Source: CAD feature listing. Evaluate the final solid. Frame: model axes, mm. A direction names the side the tool comes from. Give positions to 0.01 mm unless a question says otherwise; leave off trailing zeros. Write each loop counter-clockwise with the first axis right and the second up, starting at its lowest first coordinate (ties: lowest second). Pieces come first, ordered by that corner, then holes. Notation, with made-up numbers: (-31, 60) - (-6, 60) arc R26 ccw to (-6, 95) - close; hole circle Ø9 at (35.25, -23). An arc over 180 degrees is marked (long way). One line per question, with ' | ' between items. Start each with the question number.
(1) Access query for faces 1 (the cylindrical face through (160.406, 19.977, 33.495)), 2 (the cylindrical face through (160.406, -38.996, 0.554)), 3 (the cylindrical face through (158, 22, -29)). Directions: +Z, -Z, +X, -X, +Y, -Y. A direction counts if a zero-diameter tool reaches every point of the face in a straight line with its end or side. Return the directions, or none.
(2) Section B-B, the plane y = 0. Return loops of the section in (x, z).
(3) Section D-D, the plane x = 154. Return loops of the section in (y, z), plus the area to 3 significant figures.
(4) Section A-A, the plane z = 0. Return loops of the section in (x, y), plus the area to 3 significant figures.
(5) Ray query, line 1 (Y direction, x = 164, z = 0); line 2 (X direction, y = -5.5, z = -31); line 3 (Z direction, x = 163.5, y = -24.5). Return the intervals inside material, ascending. Write a range as [from, to].
(6) Draft query along Z for faces 4 (the cylindrical face through (160.406, 19.019, -34.048)), 5 (the flat face through (139.7, 38.02, -9.35)), 6 (the cylindrical face through (153.267, -18.922, -33.391)), 7 (the cylindrical face through (180.71, 20.76, 10.8)). Return one class per face: +Z half, -Z half, draft (parallel to the pull), parting line (faces both ways), or undercut.
(7) Section C-C, the plane z = 14.5. Return loops of the section in (x, y), plus the area to 3 significant figures.
(8) Pin query (flat end, axial travel): pin 1 (12 mm diameter, centred on x = 168.5, y = 6.5, fed in from -Z); pin 2 (1.5 mm diameter, centred on x = 144, y = 30, fed in from +Z); pin 3 (12 mm diameter, centred on x = 150, z = 16.5, fed in from -Y). Return the tip coordinate at first contact, or that it passes through.
```python
from build123d import *

# Parameters (mm, degrees)
AXIAL_HOLES_DEPTH      = 192.606080279
AXIAL_HOLES_DEPTH_BACK = 192.606080279
SKETCH2_R              = 1.65


with BuildPart() as part:
    # Axial profile (mm) → Full revolution (revolve)
    with BuildSketch(Plane.XY, mode=Mode.PRIVATE) as full_revolution_sk:
        Polygon((135.7, 36.4), (179.7, 36.4), (179.7, 23.4), (181.7, 23.4), (181.7, 39), (139.7, 39), (139.7, 43), (135.7, 43), align=None)
    revolve(full_revolution_sk.sketch.rotate(Axis((-110, 0, 0), (1, 0, 0)), 90), axis=Axis((-110, 0, 0), (1, 0, 0)))

    # Sketch2 → Axial holes (cut, two sides: drawn at the far end of the back side and taken through both)
    with BuildSketch(Plane(origin=(0, 0, 0), x_dir=(0, 0, -1), z_dir=(1, 0, 0)).offset(-AXIAL_HOLES_DEPTH_BACK)):
        with Locations(Location((0, 40, 0), (0, 0, 218.251159994))):
            Circle(SKETCH2_R)
        with Locations(Location((-34.641016151, -20, 0), (0, 0, 81.748840006))):
            Circle(SKETCH2_R)
        with Locations(Location((34.641016151, -20, 0), (0, 0, 201.748840006))):
            Circle(SKETCH2_R)
    extrude(amount=AXIAL_HOLES_DEPTH + AXIAL_HOLES_DEPTH_BACK, mode=Mode.SUBTRACT)


solid = part.part
```
Check sheet entries:
1) face 1: +Z, +X | face 2: +X, -Y | face 3: -X
2) outline: (135.7, -43) - (139.7, -43) - (139.7, -39) - (181.7, -39) - (181.7, -23.4) - (179.7, -23.4) - (179.7, -36.4) - (135.7, -36.4) - close; (135.7, 36.4) - (179.7, 36.4) - (179.7, 23.4) - (181.7, 23.4) - (181.7, 39) - (139.7, 39) - (139.7, 43) - (135.7, 43) - close
3) outline: (-20.61, -33.11) arc R1.65 cw to (-18.37, -34.4) arc R39 ccw to (38.98, -1.3) arc R1.65 cw to (38.98, 1.3) arc R39 ccw to (-18.37, 34.4) arc R1.65 cw to (-20.61, 33.11) arc R39 ccw to start; hole circle Ø72.8 at (0, 0) | area: 612 mm²
4) outline: (135.7, -43) - (139.7, -43) - (139.7, -39) - (181.7, -39) - (181.7, -23.4) - (179.7, -23.4) - (179.7, -36.4) - (135.7, -36.4) - close; (135.7, 36.4) - (179.7, 36.4) - (179.7, 23.4) - (181.7, 23.4) - (181.7, 38.35) - (135.7, 38.35) - close; (135.7, 41.65) - (139.7, 41.65) - (139.7, 43) - (135.7, 43) - close | area: 283 mm²
5) line 1: [-39, -36.4], [36.4, 38.35] | line 2: [179.7, 181.7] | line 3: [-30.34, -26.92], [26.92, 30.34]
6) face 4: -Z half | face 5: draft | face 6: undercut | face 7: undercut
7) outline: (135.7, -40.48) - (139.7, -40.48) - (139.7, -36.2) - (181.7, -36.2) - (181.7, -18.37) - (179.7, -18.37) - (179.7, -33.39) - (135.7, -33.39) - close; (135.7, 33.39) - (179.7, 33.39) - (179.7, 18.37) - (181.7, 18.37) - (181.7, 36.2) - (139.7, 36.2) - (139.7, 40.48) - (135.7, 40.48) - close | area: 353 mm²
8) pin 1: z = -39 | pin 2: z = 25.8 | pin 3: y = -37.56
